from build123d import *

# Parameters (mm, degrees)
SKETCH_1_W                   = 55
SKETCH_1_H                   = 19
SKETCH_1_R                   = 1.5
EXTRUDE_1_DEPTH              = 5
HOLE_WIZARD_M3_2_D           = 2.5
HOLE_WIZARD_M3_2_DEPTH       = 10
HOLE_WIZARD_M3_2_CSINK_D     = 3.05
HOLE_WIZARD_M3_2_CSINK_ANGLE = 90
HOLE_WIZARD_M3_2_TIP         = 0.751075774


with BuildPart() as part:
    # 草圖1 → 填料-伸長1 (new body)
    with BuildSketch(Plane.XY):
        Rectangle(SKETCH_1_W, SKETCH_1_H)
        with Locations((18, -4.5)):
            Circle(SKETCH_1_R, mode=Mode.SUBTRACT)
        with Locations((6, -4.5)):
            Circle(SKETCH_1_R, mode=Mode.SUBTRACT)
        with Locations((-6, -4.5)):
            Circle(SKETCH_1_R, mode=Mode.SUBTRACT)
        with Locations((-18, -4.5)):
            Circle(SKETCH_1_R, mode=Mode.SUBTRACT)
    extrude(amount=EXTRUDE_1_DEPTH)

    # M3 螺紋孔2
    with Locations(Plane(origin=(-24, 9.5, 2.5), x_dir=(1, 0, 0), z_dir=(0, 1, 0))):
        with Locations((0, 0), (12, 0), (24, 0), (36, 0), (48, 0)):
            CounterSinkHole(HOLE_WIZARD_M3_2_D / 2, HOLE_WIZARD_M3_2_CSINK_D / 2, depth=HOLE_WIZARD_M3_2_DEPTH, counter_sink_angle=HOLE_WIZARD_M3_2_CSINK_ANGLE)
            with Locations((0, 0, -(HOLE_WIZARD_M3_2_DEPTH + HOLE_WIZARD_M3_2_TIP / 2))):  # 118° drill point
                Cone(0, HOLE_WIZARD_M3_2_D / 2, HOLE_WIZARD_M3_2_TIP, mode=Mode.SUBTRACT)


solid = part.part
Work out the finished part from the listing and answer in its coordinate system (mm). A direction names the side the tool comes from. Round coordinates to 2 decimals unless told otherwise and drop trailing zeros. Write each loop counter-clockwise with the first axis right and the second up, starting at its lowest first coordinate (ties: lowest second). Pieces come first, ordered by that corner, then holes.
1) The mould has two halves that part along Z. Classify faces 3 (the conical face through (-0.028, -1.121, 2.285)), 4 (the cylindrical face through (16.5, -4.43, 2.46)), 5 (the flat face through (0, 0, 0)): pulls with the +Z half, pulls with the -Z half, needs draft (parallel to the pull), parting line crosses it, or undercut.
2) Given pin 1 Ø1.5 at (x, z) = (12, 2.5) entering from +Y, flat-ended and moving along its own axis, determine where the tip first touches the part or whether it passes through.
3) A cutting plane is placed at A-A (x = -6). Give the vertices of the cut face in (y, z).
4) A tool of negligible diameter and unlimited length cuts with its end or side. For faces 1 (the cylindrical face through (-25.155, 4.294, 2.979)), 2 (the flat face through (0, -9.5, 2)), from which of +Z, -Z, +X, -X, +Y, -Y can it reach the whole face along a straight path? Write none if from no direction.
5) A cutting plane is placed at B-B (y = 2.75). Give the vertices of the cut face in (x, z).
6) A cutting plane is placed at C-C (y = -3.5). Give the vertices of the cut face in (x, z), plus the area to 3 significant figures.
7) Straight lines are drawn through the part: line 1 (Z direction, x = -12, y = 5); line 2 (Y direction, x = -6, z = 2.35); line 3 (X direction, y = 8.25, z = 3.3). For each, find the intervals that lie inside material, in ascending order.
Completed:
1. face 3: undercut
1. face 4: needs draft
1. face 5: pulls with the -Z half
2. pin 1: stops at y = -0.8
3. outline: (-9.5, 0) - (-6, 0) - (-6, 5) - (-9.5, 5) - close; (-3, 0) - (9.5, 0) - (9.5, 5) - (-3, 5) - close
4. face 1: +Y
4. face 2: +Z, -Z, +X, -X, -Y
5. outline: (-27.5, 0) - (27.5, 0) - (27.5, 5) - (-27.5, 5) - close; hole circle Ø2.5 at (-24, 2.5); hole circle Ø2.5 at (-12, 2.5); hole circle Ø2.5 at (0, 2.5); hole circle Ø2.5 at (12, 2.5); hole circle Ø2.5 at (24, 2.5)
6. outline: (-27.5, 0) - (-19.12, 0) - (-19.12, 5) - (-27.5, 5) - close; (-16.88, 0) - (-7.12, 0) - (-7.12, 5) - (-16.88, 5) - close; (-4.88, 0) - (4.88, 0) - (4.88, 5) - (-4.88, 5) - close; (7.12, 0) - (16.88, 0) - (16.88, 5) - (7.12, 5) - close; (19.12, 0) - (27.5, 0) - (27.5, 5) - (19.12, 5) - close
6. area: 230 mm2
7. line 1: z = 0 to 1.25, 3.75 to 5
7. line 2: y = -9.5 to -6, -3 to 9.5
7. line 3: x = -27.5 to -24.96, -23.04 to -12.96, -11.04 to -0.96, 0.96 to 11.04, 12.96 to 23.04, 24.96 to 27.5
